Check sheet for the modelled part. Datum: model origin and axes. Units: mm. A direction names the side the tool comes from. Round coordinates to 2 decimals unless told otherwise and drop trailing zeros. Loops run counter-clockwise (first coordinate to the right, second up) from the corner with the lowest first, then second, coordinate; pieces in that order, holes last. Notation, with made-up numbers: (-4.5, -6) - (31.5, -6) arc R8 cw to (31.5, 0) - close; hole circle Ø8 at (-3, 0.5). An arc over 180 degrees is marked (long way). Return JSON: item names as keys, results as strings.
from build123d import *

# Parameters (mm, degrees)
F0_R     = 35
F0_R_2   = 1.5
F0_W     = 19.983293198
F0_H     = 32
F1_DEPTH = 2
F2_DEPTH = 4


# Not quite as in the source:
# - a feature names something its author has since deleted; it is built from what else it names


with BuildPart() as f1:
    # F0 (on Top) → F1 (new body)
    with BuildSketch(Plane.XY):
        Circle(F0_R)
        with Locations((0, -32.5)):
            Circle(F0_R_2, mode=Mode.SUBTRACT)
        with Locations((-32.5, 0)):
            Circle(F0_R_2, mode=Mode.SUBTRACT)
        with BuildLine():
            ThreePointArc((29.7321374946, 4), (29.9329594664, 2.0044793789), (30, 0))
            ThreePointArc((30, 0), (29.9329594664, -2.0044793789), (29.7321374946, -4))
            ThreePointArc((29.7321374946, -4), (21.2132034356, -21.2132034356), (4, -29.7321374946))
            ThreePointArc((4, -29.7321374946), (0, -30), (-4, -29.7321374946))
            ThreePointArc((-4, -29.7321374946), (-21.2132034356, -21.2132034356), (-29.7321374946, -4))
            ThreePointArc((-29.7321374946, -4), (-30, 0), (-29.7321374946, 4))
            ThreePointArc((-29.7321374946, 4), (-21.2132034356, 21.2132034356), (-4, 29.7321374946))
            ThreePointArc((-4, 29.7321374946), (0, 30), (4, 29.7321374946))
            ThreePointArc((4, 29.7321374946), (21.2132034356, 21.2132034356), (29.7321374946, 4))
        make_face(mode=Mode.SUBTRACT)
        with Locations((32.5, 0)):
            Circle(F0_R_2, mode=Mode.SUBTRACT)
        with Locations((0, 32.5)):
            Circle(F0_R_2, mode=Mode.SUBTRACT)
        with BuildLine():
            Line((4, 18), (4, 29.7321374946))
            ThreePointArc((4, 29.7321374946), (0, 30), (-4, 29.7321374946))
            Line((-4, 29.7321374946), (-4, 18))
            Line((-4, 18), (4, 18))
        make_face()
        with BuildLine():
            Line((-12, 4), (-29.7321374946, 4))
            ThreePointArc((-29.7321374946, 4), (-30, 0), (-29.7321374946, -4))
            Line((-29.7321374946, -4), (-12, -4))
            Line((-12, -4), (-12, 4))
        make_face()
        with BuildLine():
            ThreePointArc((-4, -29.7321374946), (0, -30), (4, -29.7321374946))
            Line((4, -29.7321374946), (4, -18))
            Line((4, -18), (-4, -18))
            Line((-4, -18), (-4, -29.7321374946))
        make_face()
        Polygon((12, -4), (12, 4), (12, 12.1005004627), (12, 18), (4, 18), (-4, 18), (-12, 18), (-12, 4), (-12, -4), (-12, -18), (-4, -18), (4, -18), (12, -18), (12, -5.151443038), align=None)
        with Locations((0.1530251862, 0.242334145)):
            Rectangle(F0_W, F0_H, mode=Mode.SUBTRACT)
        with Locations((0.1530251862, 0.242334145)):
            Rectangle(F0_W, F0_H)
        with BuildLine():
            ThreePointArc((29.7321374946, -4), (29.9329594664, -2.0044793789), (30, 0))
            ThreePointArc((30, 0), (29.9329594664, 2.0044793789), (29.7321374946, 4))
            Line((29.7321374946, 4), (12, 4))
            Line((12, 4), (12, -4))
            Line((12, -4), (29.7321374946, -4))
        make_face()
    extrude(amount=F1_DEPTH)

    # F0 (on Top) → F2 (join)
    with BuildSketch(Plane.XY):
        Polygon((12, -4), (12, 4), (12, 12.1005004627), (12, 18), (4, 18), (-4, 18), (-12, 18), (-12, 4), (-12, -4), (-12, -18), (-4, -18), (4, -18), (12, -18), (12, -5.151443038), align=None)
        with Locations((0.1530251862, 0.242334145)):
            Rectangle(F0_W, F0_H, mode=Mode.SUBTRACT)
    extrude(amount=F2_DEPTH)


solid = f1.part
Q1. Depth check by flat-ended pin: P1, Ø1, axis at x = -23.5, z = 0.5, coming from the +Y side; P2, Ø1.6, axis at y = -21, z = 1, coming from the +X side; P3, Ø1.6, axis at x = 1.5, z = 3, coming from the -Y side; P4, Ø2.5, axis at x = 0, y = -32.5, coming from the -Z side. Enter the tip coordinate at first touch or a pass-through.
Answer key:
{"P1": "stops at y = 26.38", "P2": "stops at x = 28.58", "P3": "stops at y = -18", "P4": "passes through"}
Q2. Sectioned sample at A-A (y = 0). Enter the section's corners in (x, z), plus the area to 3 significant figures.
Answer key:
{"outline": "(-35, 0) - (-34, 0) - (-34, 2) - (-35, 2) - close; (-31, 0) - (31, 0) - (31, 2) - (12, 2) - (12, 4) - (10.14, 4) - (10.14, 2) - (-9.84, 2) - (-9.84, 4) - (-12, 4) - (-12, 2) - (-31, 2) - close; (34, 0) - (35, 0) - (35, 2) - (34, 2) - close", "area": "136 mm²"}
Q3. Tool access check on faces 1 (the face through (-21, -4, 1)), 2 (the face through (0.2, 18, 2.4)). Record the directions out of +Z, -Z, +X, -X, +Y, -Y that give a thin tool (end or side, any length) a straight path to the whole face; none if there is none.
Answer key:
{"face 1": "+Z, -Z", "face 2": "+Z"}
Q4. Sectioned sample at B-B (z = 2.9). Enter the section's corners in (x, y).
Answer key:
{"outline": "(-12, -18) - (12, -18) - (12, 18) - (-12, 18) - close; hole (-9.84, -15.76) - (10.14, -15.76) - (10.14, 16.24) - (-9.84, 16.24) - close"}
Q5. Sectioned sample at C-C (x = -13.5). Enter the section's corners in (y, z), plus the area to 3 significant figures.
Answer key:
{"outline": "(-32.29, 0) - (-26.79, 0) - (-26.79, 2) - (-32.29, 2) - close; (-4, 0) - (4, 0) - (4, 2) - (-4, 2) - close; (26.79, 0) - (32.29, 0) - (32.29, 2) - (26.79, 2) - close", "area": "38.0 mm²"}
Q6. Sectioned sample at D-D (y = -32.5). Enter the section's corners in (x, z).
Answer key:
{"outline": "(-12.99, 0) - (-1.5, 0) - (-1.5, 2) - (-12.99, 2) - close; (1.5, 0) - (12.99, 0) - (12.99, 2) - (1.5, 2) - close"}
Q7. Scan lines: probe 1 along Y at (x, z) = (0, 1.3); probe 2 along X at (y, z) = (9.5, 3.4); probe 3 along Y at (x, z) = (-16.5, 1.5). Record each from-to range of solid material in increasing order. Write a range as [from, to].
Answer key:
{"probe 1": "y = [-35, -34], [-31, 31], [34, 35]", "probe 2": "x = [-12, -9.84], [10.14, 12]", "probe 3": "y = [-30.87, -25.05], [-4, 4], [25.05, 30.87]"}
Q8. Draft check along X on faces 3 (the face through (4, -24, 1)), 4 (the face through (-21.406, 21.019, 0.986)), 5 (the face through (-28, -21, 1)). Enter one of: released by +X, released by -X, zero draft, split by the parting line, or undercut.
Answer key:
{"face 3": "undercut", "face 4": "undercut", "face 5": "split by the parting line"}
